Read the model definition and answer for the solid it produces. Units are mm, in the model's axes. Coordinates: 2 decimals unless noted, no trailing zeros. Loops run counter-clockwise (first coordinate to the right, second up) from the corner with the lowest first, then second, coordinate; pieces in that order, holes last. Notation, with made-up numbers: (30.5, 79) - (54.5, 79) arc R15 ccw to (54.5, 88) - close; hole circle Ø1 at (55.25, 42.25). An arc over 180 degrees is marked (long way). Use one line per item in the form item = value.
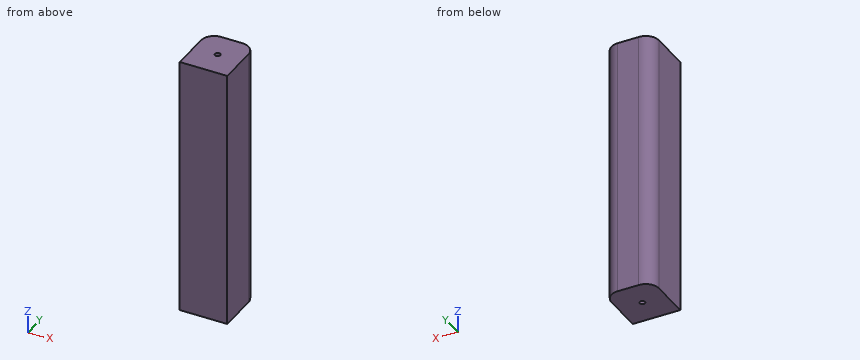
from build123d import *

# Parameters (mm, degrees)
EXTRUDE_1_DEPTH     = 99
SKETCH_2_R          = 1
CUT_EXTRUDE_1_DEPTH = 5
CUT_EXTRUDE_START   = -5
SKETCH_3_R          = 1
CUT_EXTRUDE_2_DEPTH = 5


with BuildPart() as part:
    # 草图1 → 凸台-拉伸1 (new body)
    with BuildSketch(Plane.XY):
        with BuildLine():
            Line((-4, 10), (4, 10))
            ThreePointArc((4, 10), (7.535533906, 8.535533906), (9, 5))
            Line((9, 5), (9, -10))
            Line((9, -10), (-9, -10))
            Line((-9, -10), (-9, 5))
            ThreePointArc((-9, 5), (-7.535533906, 8.535533906), (-4, 10))
        make_face()
    extrude(amount=EXTRUDE_1_DEPTH)

    # 草图2 → 切除-拉伸1 (cut)
    with BuildSketch(Plane.XY.offset(99)):
        Circle(SKETCH_2_R)
    extrude(amount=-CUT_EXTRUDE_1_DEPTH, mode=Mode.SUBTRACT)

    # 草图3 → 切除-拉伸2 (cut)
    with BuildSketch(Plane(origin=(0, 0, 0), x_dir=(-1, 0, 0), z_dir=(0, 0, -1)).offset(CUT_EXTRUDE_START)):
        with Locations(Location((0, 0, 0), (0, 0, 180))):
            Circle(SKETCH_3_R)
    extrude(amount=CUT_EXTRUDE_2_DEPTH, mode=Mode.SUBTRACT)


solid = part.part
Item 1: Find the intervals of material crossed by L1, parallel to Y at x = 0, z = 97.8; L2, parallel to Y at x = 8, z = 51; L3, parallel to Y at x = 7.25, z = 83, in increasing order.
Results below:
L1 = -10 to -1, 1 to 10
L2 = -10 to 8
L3 = -10 to 8.8
Item 2: The part is cut by section A-A on z = 21. Give the vertices of the cut face in (x, y), plus the area to 3 significant figures.
Results below:
outline = (-9, -10) - (9, -10) - (9, 5) arc R5 ccw to (4, 10) - (-4, 10) arc R5 ccw to (-9, 5) - close
area = 349 mm²
Item 3: The part is cut by section B-B on x = 6. Give the vertices of the cut face in (y, z), plus the area to 3 significant figures.
Results below:
outline = (-10, 0) - (9.58, 0) - (9.58, 99) - (-10, 99) - close
area = 1,940 mm²
Item 4: Each of these flat-tipped pins is pushed along its axis until it touches: P1, Ø1.6, axis at x = 0, y = 0, coming from the -Z side; P2, Ø1.5, axis at y = 6, z = 53.5, coming from the -X side. Where does it stop, or does it pass through?
Results below:
P1 = 5
P2 = -8.99
